The figure shows three views and two pictorial views of one solid part (mm, origin at its lowest corner). Answer the questions. A direction names the side the tool comes from. Round coordinates to 2 decimals unless told otherwise and drop trailing zeros. Order: outer loops, then holes, each group sorted by start corner. A loop starts at its lowest first (then second) coordinate and runs counter-clockwise, first axis right, second up. Notation, with made-up numbers: (61.5, 58.25) -> (95.5, 58.25) arc R31 cw to (95.5, 92.25) -> close; hole circle Ø1 at (43.5, 75). An arc over 180 degrees is marked (long way). One line per item, written item: value. Start each with the question number.
1. Section A-A (x = 16) is taken. Give the vertices of the cut face in (y, z), then the cut area to 3 significant figures.
2. Section B-B (z = 16) is taken. Give the vertices of the cut face in (x, y), then the cut area to 3 significant figures.
3. The mould has two halves that part along Y. Classify the marked faces 1, 2 and 3: released by +Y, released by -Y, zero draft, split by the parting line, or undercut.
4. For the marked faces 4 and 5, determine the directions among +Z, -Z, +X, -X, +Y, -Y from which every point of the face is accessible in a straight line to the end or side of a thin tool.
5. Section D-D (y = 14.25) is taken. Give the vertices of the cut face in (x, z).
6. Flat-ended cylindrical pins translate along their axes: pin 1 Ø2.5 at (x, z) = (4, 16) entering from -Y; pin 2 Ø2.5 at (y, z) = (7.5, 10) entering from -X; pin 3 Ø2.5 at (y, z) = (7.5, 10) entering from +X. Find the tip coordinate at first contact, or state that the pin passes through.
7. Section C-C (x = 4) is taken. Give the vertices of the cut face in (y, z).
8. Consider line 1 (Z direction, x = 4, y = 1.7); line 2 (Z direction, x = 3, y = 9.75). Determine where each line is inside the solid, lowest interval first.
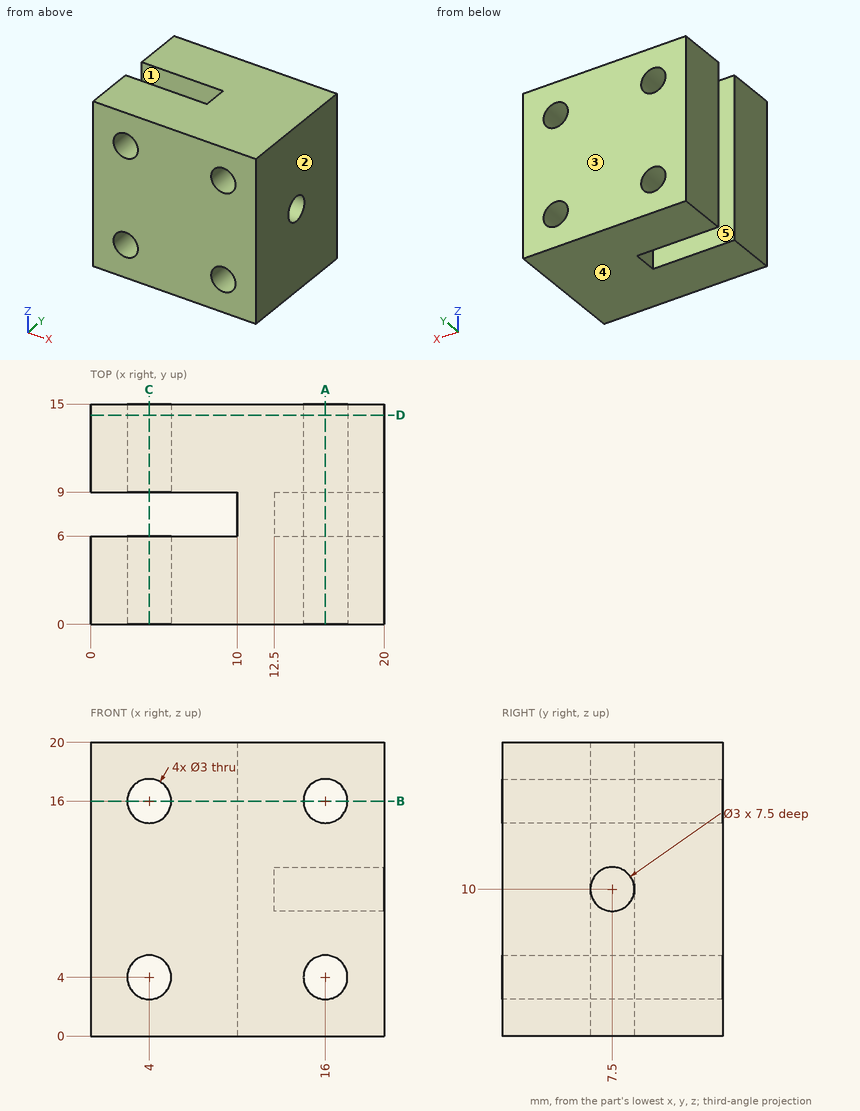
Answer:
1. outline: (0, 0) -> (15, 0) -> (15, 2.5) -> (0, 2.5) -> close; (0, 5.5) -> (15, 5.5) -> (15, 14.5) -> (0, 14.5) -> close; (0, 17.5) -> (15, 17.5) -> (15, 20) -> (0, 20) -> close; hole circle Ø3 at (7.5, 10)
1. area: 203 mm^2
2. outline: (0, 0) -> (2.5, 0) -> (2.5, 6) -> (0, 6) -> close; (0, 9) -> (2.5, 9) -> (2.5, 15) -> (0, 15) -> close; (5.5, 0) -> (14.5, 0) -> (14.5, 15) -> (5.5, 15) -> (5.5, 9) -> (10, 9) -> (10, 6) -> (5.5, 6) -> close; (17.5, 0) -> (20, 0) -> (20, 15) -> (17.5, 15) -> close
2. area: 189 mm^2
3. face 1: undercut
3. face 2: zero draft
3. face 3: released by +Y
4. face 4: -Z, +X, -X, +Y, -Y
4. face 5: +Z, -Z, -X
5. outline: (0, 0) -> (20, 0) -> (20, 20) -> (0, 20) -> close; hole circle Ø3 at (4, 4); hole circle Ø3 at (4, 16); hole circle Ø3 at (16, 4); hole circle Ø3 at (16, 16)
6. pin 1: through
6. pin 2: x = 10
6. pin 3: x = 12.5
7. outline: (0, 0) -> (6, 0) -> (6, 2.5) -> (0, 2.5) -> close; (0, 5.5) -> (6, 5.5) -> (6, 14.5) -> (0, 14.5) -> close; (0, 17.5) -> (6, 17.5) -> (6, 20) -> (0, 20) -> close; (9, 0) -> (15, 0) -> (15, 2.5) -> (9, 2.5) -> close; (9, 5.5) -> (15, 5.5) -> (15, 14.5) -> (9, 14.5) -> close; (9, 17.5) -> (15, 17.5) -> (15, 20) -> (9, 20) -> close
8. line 1: 0 to 2.5, 5.5 to 14.5, 17.5 to 20
8. line 2: 0 to 2.88, 5.12 to 14.88, 17.12 to 20
